Build history of the part. All positions in model axes, mm. A direction names the side the tool comes from. Give positions to 0.01 mm unless a question says otherwise; leave off trailing zeros. Write each loop counter-clockwise with the first axis right and the second up, starting at its lowest first coordinate (ties: lowest second). Pieces come first, ordered by that corner, then holes. Notation, with made-up numbers: (26.25, 24.25) -> (65.25, 24.25) arc R26 cw to (65.25, 61.25) -> close; hole circle Ø2 at (-1, 87). An arc over 180 degrees is marked (long way). One line per question, with ' | ' between items. Start each with the question number.
(1) Pin check, flat tips, straight feed: P1, Ø4, axis at x = -30, z = -46, coming from the -Y side; P2, Ø1, axis at y = 5.5, z = -61, coming from the -X side; P3, Ø1.5, axis at y = 2, z = 11, coming from the +X side. Stop position of each tip, or through.
(2) Band-saw the part on C-C, the plane z = 69.85. Give the cut face in (x, y) (3 decimals), and give its area (3 significant figures).
(3) Band-saw the part on A-A, the plane x = -41.5. Give the cut face in (y, z), and give its area (3 significant figures).
(4) Band-saw the part on D-D, the plane y = 3.5. Count the separate pieces of the cut face and the enclosed holes in it, and give its area (3 significant figures).
(5) Band-saw the part on B-B, the plane x = 0. Give the cut face in (y, z) (3 decimals), and give its area (3 significant figures).
(6) Tool access for faces 1 (the cylindrical face through (-11.22, 3.13, -70.21)), 2 (the flat face through (13, 3, 58.018)): list every direction of +Z, -Z, +X, -X, +Y, -Y with a clear straight run to the whole face (end or side of a thin tool).
(7) Pull direction Z, two halves, no side cores. Call faces 3 (the flat face through (13, 3, -58.018)), 4 (the cylindrical face through (-0.14, 3.13, 66.59)), 5 (the flat face through (22.225, 3, 72)), 6 (the flat face through (9, 3, 79.375)): released by +Z, released by -Z, zero draft, split by the parting line, or undercut.
(8) Drill centre lines: probe 1 along Z at (x, y) = (10, 5) (3 decimals); probe 2 along Z at (x, y) = (6.5, 4) (3 decimals); probe 3 along X at (y, z) = (1.75, -69.85) (3 decimals). Where is each one in solid material? Low to high. Write a range as from..to.
from build123d import *

# Parameters (mm, degrees)
SKETCH1_R                = 69.85
SKETCH1_R_2              = 56.35625
BOSS_EXTRUDE1_DEPTH      = 6.35
SKETCH5_W                = 19.05
SKETCH5_H                = 15.875
BOSS_EXTRUDE2_DEPTH      = 6.35
FILLET1_R                = 6.35
CIRPATTERN2_COUNT        = 3
CIRPATTERN2_ANGLE        = 180
FILLET1_OF_CIRPATTERN2_R = 6.35
SKETCH11_R               = 3.2639
CUT_EXTRUDE2_DEPTH       = 113.432663181
CIRPATTERN3_COUNT        = 3
CIRPATTERN3_ANGLE        = 180
CUT_EXTRUDE4_DEPTH       = 113.432663181
FILLET8_R                = 6.35
SKETCH22_W               = 21.356989326
SKETCH22_H               = 6.35
BOSS_EXTRUDE3_DEPTH      = 12.7
SKETCH23_R               = 2.15265
CUT_EXTRUDE5_DEPTH       = 113.432663328
FILLET11_R               = 6.35


with BuildPart() as part:
    # Sketch1 → Boss-Extrude1 (new body)
    with BuildSketch(Plane(origin=(0, 0, 0), x_dir=(1, 0, 0), z_dir=(0, 1, 0))):
        with Locations(Location((0, 0, 0), (0, 0, 270))):
            Circle(SKETCH1_R)
        with Locations(Location((0, 0, 0), (0, 0, 270))):
            Circle(SKETCH1_R_2, mode=Mode.SUBTRACT)
    extrude(amount=BOSS_EXTRUDE1_DEPTH)

    # Sketch5 → Boss-Extrude2 (add)
    with BuildSketch(Plane(origin=(0, 6.35, 0), x_dir=(1, 0, 0), z_dir=(0, 1, 0))):
        with Locations((0, 71.4375)):
            Rectangle(SKETCH5_W, SKETCH5_H)
    boss_extrude2 = extrude(amount=-BOSS_EXTRUDE2_DEPTH)

    # Fillet1
    fillet1_edges = [part.edges().sort_by_distance(p)[0] for p in [
        (9.525, 3.175, -69.197520729),
        (-9.525, 3.175, -69.197520729),
    ]]
    fillet(fillet1_edges, radius=FILLET1_R)

    # CirPattern2: Boss-Extrude2 ×3 about axis
    cirpattern2_axis = Axis((0, 0, 0), (0, 1, 0))
    for i in range(1, CIRPATTERN2_COUNT):
        add(boss_extrude2.rotate(cirpattern2_axis, i * CIRPATTERN2_ANGLE / (CIRPATTERN2_COUNT - 1)))

    # Fillet1 of CirPattern2
    fillet1_of_cirpattern2_edges = [part.edges().sort_by_distance(p)[0] for p in [
        (-69.197520729, 3.175, -9.525),
        (-69.197520729, 3.175, 9.525),
        (-9.525, 3.175, 69.197520729),
        (9.525, 3.175, 69.197520729),
    ]]
    fillet(fillet1_of_cirpattern2_edges, radius=FILLET1_OF_CIRPATTERN2_R)

    # Sketch11 → Cut-Extrude2 (cut, through all)
    with BuildSketch(Plane.XZ):
        with Locations(Location((0, -69.85, 0), (0, 0, 270))):
            Circle(SKETCH11_R)
    cut_extrude2 = extrude(amount=-CUT_EXTRUDE2_DEPTH, mode=Mode.SUBTRACT)

    # CirPattern3: Cut-Extrude2 ×3 about axis
    cirpattern3_axis = Axis((0, 0, 0), (0, 1, 0))
    for i in range(1, CIRPATTERN3_COUNT):
        add(cut_extrude2.rotate(cirpattern3_axis, i * CIRPATTERN3_ANGLE / (CIRPATTERN3_COUNT - 1)), mode=Mode.SUBTRACT)

    # Sketch14 → Cut-Extrude4 (cut, through all)
    with BuildSketch(Plane(origin=(0, 6.35, 0), x_dir=(1, 0, 0), z_dir=(0, 1, 0))):
        Polygon((76.141203704, 74.528010674), (76.141203704, -74.528010674), (9.525, -74.528010674), (9.525, -58.018010674), (-10.795, -55.312700974), (-10.795, 55.312700974), (9.525, 58.018010674), (9.525, 74.528010674), align=None)
    extrude(amount=-CUT_EXTRUDE4_DEPTH, mode=Mode.SUBTRACT)

    # Fillet8
    fillet8_edges = [part.edges().sort_by_distance(p)[0] for p in [
        (-9.525, 3.175, 79.375),
        (-79.375, 3.175, 9.525),
        (-79.375, 3.175, -9.525),
        (-9.525, 3.175, -79.375),
    ]]
    fillet(fillet8_edges, radius=FILLET8_R)

    # Sketch22 → Boss-Extrude3 (add)
    with BuildSketch(Plane(origin=(9.525, 0, 0), x_dir=(0, 0, -1), z_dir=(1, 0, 0))):
        with Locations((68.696505337, 3.175)):
            Rectangle(SKETCH22_W, SKETCH22_H)
    boss_extrude3 = extrude(amount=BOSS_EXTRUDE3_DEPTH)

    # Sketch23 → Cut-Extrude5 (cut, through all)
    with BuildSketch(Plane(origin=(0, 6.35, 0), x_dir=(1, 0, 0), z_dir=(0, 1, 0))):
        with Locations(Location((15.7226, 64.77, 0), (0, 0, 270))):
            Circle(SKETCH23_R)
    cut_extrude5 = extrude(amount=-CUT_EXTRUDE5_DEPTH, mode=Mode.SUBTRACT)

    # Mirror1: Boss-Extrude3, Cut-Extrude5 across plane
    add(boss_extrude3.mirror(Plane.XY))
    add(cut_extrude5.mirror(Plane.XY), mode=Mode.SUBTRACT)

    # Fillet11
    fillet11_edges = [part.edges().sort_by_distance(p)[0] for p in [
        (22.225, 3.175, -58.018010674),
        (22.225, 3.175, 58.018010674),
    ]]
    fillet(fillet11_edges, radius=FILLET11_R)


solid = part.part
Results:
1) P1: stops at y = 0 | P2: stops at x = -34.91 | P3: stops at x = -55.12
2) outline: (-11.581, 0) -> (-3.264, 0) -> (-3.264, 6.35) -> (-11.581, 6.35) -> close; (3.264, 0) -> (22.225, 0) -> (22.225, 6.35) -> (3.264, 6.35) -> close | area: 173 mm²
3) outline: (0, -56.19) -> (6.35, -56.19) -> (6.35, -38.13) -> (0, -38.13) -> close; (0, 38.13) -> (6.35, 38.13) -> (6.35, 56.19) -> (0, 56.19) -> close | area: 229 mm²
4) separate pieces: 1 | enclosed holes: 5 | area: 3,850 mm²
5) outline: (0, -79.375) -> (6.35, -79.375) -> (6.35, -73.114) -> (0, -73.114) -> close; (0, -66.586) -> (6.35, -66.586) -> (6.35, -56.75) -> (0, -56.75) -> close; (0, 56.75) -> (6.35, 56.75) -> (6.35, 66.586) -> (0, 66.586) -> close; (0, 73.114) -> (6.35, 73.114) -> (6.35, 79.375) -> (0, 79.375) -> close | area: 204 mm²
6) face 1: -Z, -X, +Y, -Y | face 2: +X, +Y, -Y
7) face 3: undercut | face 4: undercut | face 5: zero draft | face 6: released by +Z
8) probe 1: z = -79.375..-58.018, 58.018..79.375 | probe 2: z = -79.375..-57.615, 57.615..79.375 | probe 3: x = -11.581..-3.264, 3.264..22.225
